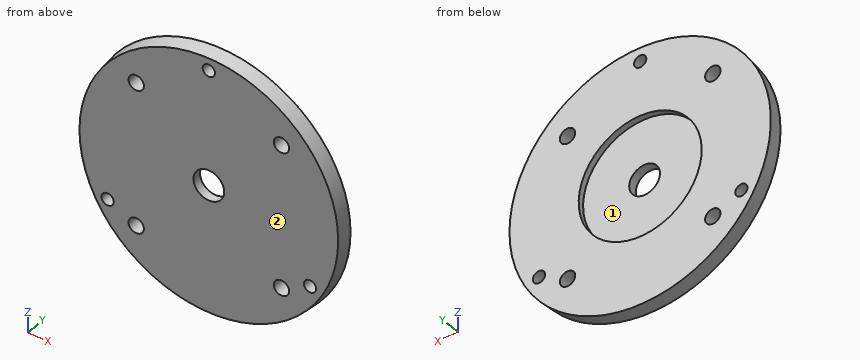
from build123d import *

# Parameters (mm, degrees)
SKETCH1_R           = 42.5
BOSS_EXTRUDE1_DEPTH = 5
BOSS_EXTRUDE1_DRAFT = -5
SKETCH2_R           = 2.5
SKETCH2_R_2         = 5
CUT_EXTRUDE2_DEPTH  = 61.311690409
SKETCH3_R           = 20
CUT_EXTRUDE3_DEPTH  = 2
SKETCH5_R           = 2
CUT_EXTRUDE4_DEPTH  = 5


with BuildPart() as part:
    # Sketch1 → Boss-Extrude1 (with draft: the straight prism first)
    with BuildSketch(Plane(origin=(0, 0, 0), x_dir=(1, 0, 0), z_dir=(0, 1, 0))):
        Circle(SKETCH1_R)
    extrude(amount=-BOSS_EXTRUDE1_DEPTH)
    # Boss-Extrude1: the draft: its side faces are tilted about the plane it starts from
    boss_extrude1_sides = [part.faces().sort_by_distance(p)[0] for p in [
        (-42.5, -2.5, 0),
    ]]
    draft(boss_extrude1_sides, Plane(origin=(0, 0, 0), x_dir=(1, 0, 0), z_dir=(0, 1, 0)), BOSS_EXTRUDE1_DRAFT)

    # Sketch2 → Cut-Extrude2 (cut, through all)
    with BuildSketch(Plane(origin=(0, 0, 0), x_dir=(1, 0, 0), z_dir=(0, 1, 0))):
        with Locations(Location((23.62, 23.62, 0), (0, 0, 270))):
            Circle(SKETCH2_R)
        with Locations(Location((23.62, -23.62, 0), (0, 0, 270))):
            Circle(SKETCH2_R)
        with Locations(Location((-23.62, -23.62, 0), (0, 0, 270))):
            Circle(SKETCH2_R)
        with Locations(Location((-23.62, 23.62, 0), (0, 0, 270))):
            Circle(SKETCH2_R)
        with Locations(Location((0, 0, 0), (0, 0, 270))):
            Circle(SKETCH2_R_2)
    extrude(amount=-CUT_EXTRUDE2_DEPTH, mode=Mode.SUBTRACT)

    # Sketch3 → Cut-Extrude3 (cut)
    with BuildSketch(Plane(origin=(0, 0, 0), x_dir=(1, 0, 0), z_dir=(0, 1, 0))):
        with Locations(Location((0, 0, 0), (0, 0, 270))):
            Circle(SKETCH3_R)
    extrude(amount=-CUT_EXTRUDE3_DEPTH, mode=Mode.SUBTRACT)

    # Sketch5 → Cut-Extrude4 (cut)
    with BuildSketch(Plane(origin=(0, 0, 0), x_dir=(1, 0, 0), z_dir=(0, 1, 0))):
        with Locations(Location((0, -38, 0), (0, 0, 270))):
            Circle(SKETCH5_R)
        with Locations(Location((-32.908965344, 19, 0), (0, 0, 270))):
            Circle(SKETCH5_R)
        with Locations(Location((32.908965344, 19, 0), (0, 0, 270))):
            Circle(SKETCH5_R)
    extrude(amount=-CUT_EXTRUDE4_DEPTH, mode=Mode.SUBTRACT)


solid = part.part
Geometry check sheet. Reference: the model listing, model coordinates, mm. Face numbers are marked on the shaded views. Give positions to 0.01 mm unless a question says otherwise; leave off trailing zeros. Write each loop counter-clockwise with the first axis right and the second up, starting at its lowest first coordinate (ties: lowest second). Pieces come first, ordered by that corner, then holes.
1) Cross-section at A-A (z = 0). Record the boundary of the cut face in (x, y), plus the area to 3 significant figures.
Values follow:
outline: (-42.5, 0) - (-42.06, -5) - (-5, -5) - (-5, -2) - (-20, -2) - (-20, 0) - close; (5, -5) - (42.06, -5) - (42.5, 0) - (20, 0) - (20, -2) - (5, -2) - close
area: 313 mm2
2) Cross-section at B-B (x = 0). Record the boundary of the cut face in (y, z), plus the area to 3 significant figures.
Values follow:
outline: (-5, -42.06) - (0, -42.5) - (0, -20) - (-2, -20) - (-2, -5) - (-5, -5) - close; (-5, 5) - (-2, 5) - (-2, 20) - (0, 20) - (0, 36) - (-5, 36) - close; (-5, 40) - (0, 40) - (0, 42.5) - (-5, 42.06) - close
area: 293 mm2
3) Cross-section at C-C (y = -0.75). Count the separate pieces of the cut face and the enclosed holes in it, plus the area to 3 significant figures.
Values follow:
separate pieces: 1
enclosed holes: 8
area: 4,280 mm2
4) Thickness scan on line 1 (X direction, y = -1.3, z = -25.5); line 2 (X direction, y = -1.8, z = 23.62); line 3 (X direction, y = -1.6, z = 1.5). Record the ranges inside material, lowest first.
Values follow:
line 1: x = -33.86 to -25.27, -21.97 to 21.97, 25.27 to 33.86
line 2: x = -35.14 to -26.12, -21.12 to 21.12, 26.12 to 35.14
line 3: x = -42.33 to -19.94, 19.94 to 42.33
5) Go/stop test with flat-tipped pins: pin 1 Ø2 at (y, z) = (-4, 3) entering from -X; pin 2 Ø11.5 at (x, z) = (0, 0) entering from +Y; pin 3 Ø1 at (y, z) = (-4, 3) entering from -X. Record where each tip stops, or that it passes through.
Values follow:
pin 1: stops at x = -42.15
pin 2: stops at y = -2
pin 3: stops at x = -42.1
6) Release check for a two-part mould opening along Z. For the marked faces 1 and 2 record: released by +Z, released by -Z, zero draft, split by the parting line, or undercut.
Values follow:
face 1: undercut
face 2: zero draft
